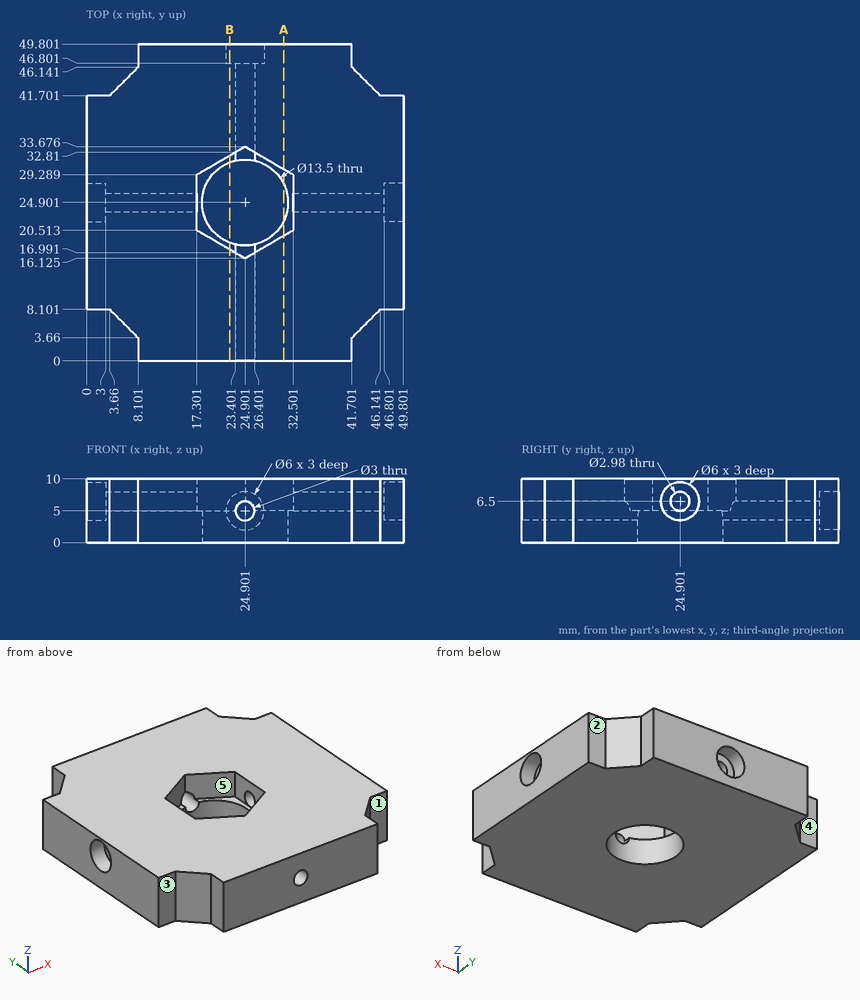
Answer from the drawing. Dimensions are ordinates in mm from the lowest x, y and z of the part. A direction names the side the tool comes from. Give positions to 0.01 mm unless a question says otherwise; leave off trailing zeros. Order: outer loops, then holes, each group sorted by start corner. A loop starts at its lowest first (then second) coordinate and runs counter-clockwise, first axis right, second up.
(1) Find section A-A (x = 31). Give the vertices of the cut face in (y, z) (1 decimal).
(2) Find section B-B (x = 22.5). Give the vertices of the cut face in (y, z).
(3) Given pin 1 (4 mm diameter, centred on x = 24.9, z = 5, fed in from +Y); pin 2 (3 mm diameter, centred on y = 25, z = 5.5, fed in from +X); pin 3 (4 mm diameter, centred on y = 47.5, z = 2.5, fed in from -X), each flat-ended and moving along its own axis, determine where each tip first touches the part or whether it passes through.
(4) For the marked faces 1, 2, 3, 4 and 5, determine the directions among +Z, -Z, +X, -X, +Y, -Y from which every point of the face is accessible in a straight line to the end or side of a thin tool.
(5) Straight lines are drawn through the part: L1, parallel to Y at x = 47.7, z = 6.5; L2, parallel to X at y = 41.5, z = 4.75. For each, find the intervals that lie inside material, in ascending order.
Result sheet:
1. outline: (0, 0) - (22, 0) - (22, 5) - (19.6, 5) - (19.6, 10) - (0, 10) - close; (27.8, 0) - (49.8, 0) - (49.8, 10) - (30.2, 10) - (30.2, 5) - (27.8, 5) - close
2. outline: (0, 0) - (18.59, 0) - (18.59, 5) - (17.51, 5) - (17.51, 10) - (0, 10) - close; (31.21, 0) - (49.8, 0) - (49.8, 3.2) - (46.8, 3.2) - (46.8, 6.8) - (49.8, 6.8) - (49.8, 10) - (32.29, 10) - (32.29, 5) - (31.21, 5) - close
3. pin 1: stops at y = 46.8
3. pin 2: stops at x = 46.8
3. pin 3: stops at x = 7.46
4. face 1: +Z, -Z, +X, -Y
4. face 2: +Z, -Z, +X, +Y
4. face 3: +Z, -Z, -X, -Y
4. face 4: +Z, -Z, -X, +Y
4. face 5: +Z
5. L1: y = 8.1 to 21.9, 27.9 to 41.7
5. L2: x = 0 to 23.42, 26.38 to 49.8
